Could you check a few things on this model? Use its own coordinates, in mm. A direction names the side the tool comes from. Coordinates: 2 decimals unless noted, no trailing zeros. Loops run counter-clockwise (first coordinate to the right, second up) from the corner with the lowest first, then second, coordinate; pieces in that order, holes last.
1) Imagine slicing it at D-D on z = 58. Please give me the cut outline in (x, y), plus the area to 3 significant figures.
2) Imagine slicing it at A-A on x = 0. Please give me the cut outline in (y, z), plus the area to 3 significant figures.
3) If I drill on line 1 along Y through (x, z) = (0, 39); line 2 along X through (y, z) = (5.5, 28.5); line 3 along Y through (x, z) = (21.5, 21), over which ranges is the centre line in solid material (lowest first)?
4) For faces 4 (the face through (42.397, 13.352, 32.017)), 5 (the face through (0, 0, 63.5)), which set-ups out of +Z, -Z, +X, -X, +Y, -Y let a thin tool reach every point of the face, with its end or its side?
5) Will these pins go through, and if not, where does the flat tip stop? P1, Ø10, axis at x = -24, z = 53, coming from the -Y side; P2, Ø1, axis at x = -7, z = 53.5, coming from the -Y side; P3, Ø6, axis at y = -42, z = 42.5, coming from the +X side.
6) Imagine slicing it at B-B on z = 39. Please give me the cut outline in (x, y), plus the area to 3 significant figures.
7) Thinking about a two-plate mould opening in Y: for faces 1 (the face through (-60.47, -46.367, 31.306)), 2 (the face through (-25.69, -19.69, 62.88)), 3 (the face through (-29, 57, 63.5)), which applies, released by +Y, released by -Y, zero draft, split by the parting line, or undercut?
```python
from build123d import *

# Parameters (mm, degrees)
F0_R     = 76.2
F1_DEPTH = 63.5
F2_R     = 50.8
F2_R_2   = 44.45
F3_DEPTH = 50.8
F4_SIZE  = 12.7


with BuildPart() as f1:
    # F0 (on Top) → F1 (new body)
    with BuildSketch(Plane.XY):
        Circle(F0_R)
    extrude(amount=F1_DEPTH)

    # F2 (on face) → F3 (cut)
    with BuildSketch(Plane.XY.offset(63.5)):
        Circle(F2_R)
        Circle(F2_R_2, mode=Mode.SUBTRACT)
    extrude(amount=-F3_DEPTH, mode=Mode.SUBTRACT)

    # F4
    f4_edges = [f1.edges().sort_by_distance(p)[0] for p in [
        (-50.8, 0, 63.5),
        (-44.45, 0, 63.5),
    ]]
    chamfer(f4_edges, length=F4_SIZE)


solid = f1.part
```
Filled in:
1. outline: circle Ø152.4 at (0, 0); circle Ø74.5 at (0, 0); hole circle Ø116 at (0, 0)
1. area: 12,000 mm2
2. outline: (-76.2, 0) - (76.2, 0) - (76.2, 63.5) - (63.5, 63.5) - (50.8, 50.8) - (50.8, 12.7) - (44.45, 12.7) - (44.45, 50.8) - (31.75, 63.5) - (-31.75, 63.5) - (-44.45, 50.8) - (-44.45, 12.7) - (-50.8, 12.7) - (-50.8, 50.8) - (-63.5, 63.5) - (-76.2, 63.5) - close
2. area: 8,710 mm2
3. line 1: y = -76.2 to -50.8, -44.45 to 44.45, 50.8 to 76.2
3. line 2: x = -76 to -50.5, -44.11 to 44.11, 50.5 to 76
3. line 3: y = -73.1 to -46.03, -38.9 to 38.9, 46.03 to 73.1
4. face 4: +Z
4. face 5: +Z, +X, -X, +Y, -Y
5. P1: stops at y = -73.79
5. P2: stops at y = -75.92
5. P3: stops at x = 65.46
6. outline: circle Ø152.4 at (0, 0); circle Ø88.9 at (0, 0); hole circle Ø101.6 at (0, 0)
6. area: 16,300 mm2
7. face 1: split by the parting line
7. face 2: undercut
7. face 3: zero draft
